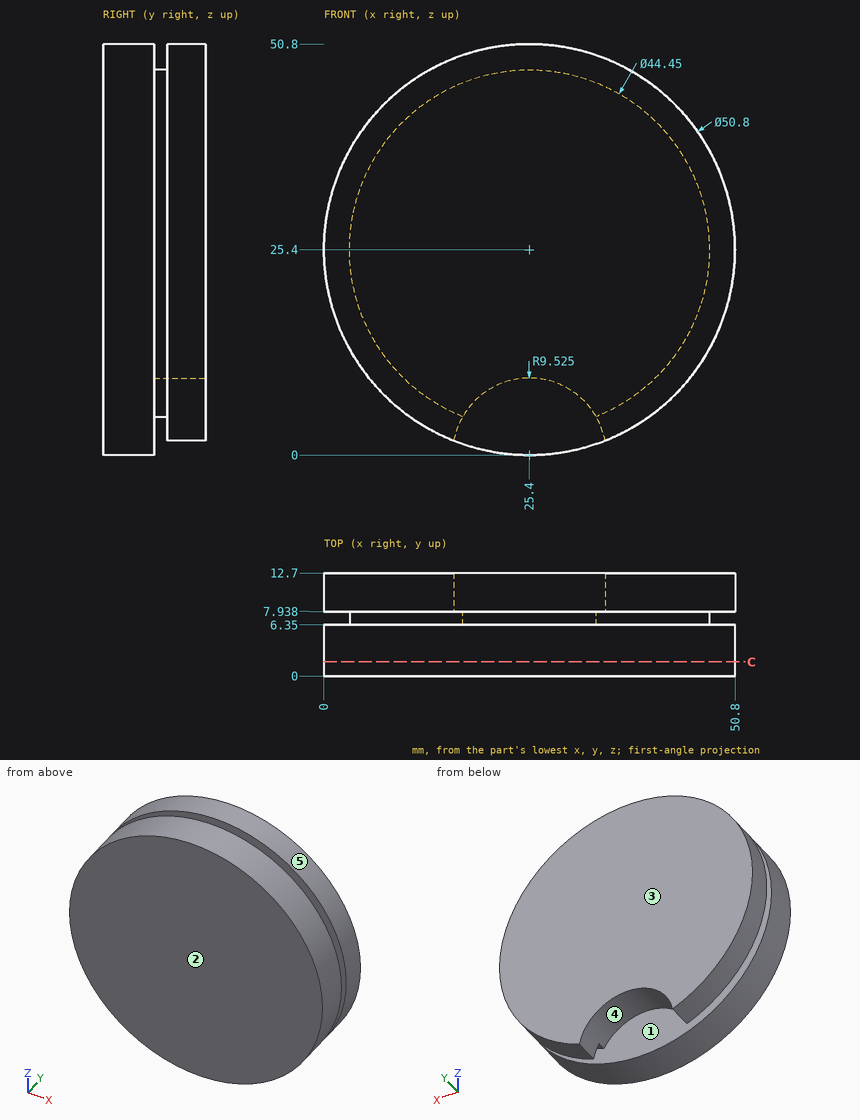
Geometry check sheet. Reference: drawing and pictorial views, mm from the part's lowest x, y, z. A direction names the side the tool comes from. Give positions to 0.01 mm unless a question says otherwise; leave off trailing zeros. Loops run counter-clockwise (first coordinate to the right, second up) from the corner with the lowest first, then second, coordinate; pieces in that order, holes last. Notation, with made-up numbers: M -26,40.25 L -9,40.25 A31 cw -9,68.25 Z; hole C 37,-25.75 d5. An arc over 180 degrees is marked long. One line per question, with ' | ' between items.
Item 1: Thickness scan on line 1 (Y direction, x = 19, z = 47); line 2 (Y direction, x = 22, z = 2); line 3 (Z direction, x = 44.5, y = 9.5) (1 decimal). Record the ranges inside material, lowest first. Write a range as [from, to].
Completed:
line 1: y = [0, 6.35], [7.94, 12.7] | line 2: y = [0, 6.35] | line 3: z = [8.7, 42.1]
Item 2: Draft check along X on the marked faces 3, 4 and 5. Enter one of: +X half, -X half, draft (parallel to the pull), parting line (faces both ways), or undercut.
Completed:
face 3: draft | face 4: undercut | face 5: parting line
Item 3: Tool access check on the marked faces 1 and 2. Record the directions out of +Z, -Z, +X, -X, +Y, -Y that give a thin tool (end or side, any length) a straight path to the whole face; none if there is none.
Completed:
face 1: none | face 2: +Z, -Z, +X, -X, -Y
Item 4: Depth check by flat-ended pin: P1, Ø1, axis at y = 4, z = 16.5, coming from the -X side; P2, Ø3, axis at y = 5.5, z = 20, coming from the +X side; P3, Ø3, axis at y = 3, z = 36, coming from the +X side (1 decimal). Enter the tip coordinate at first touch or a pass-through.
Completed:
P1: stops at x = 1.43 | P2: stops at x = 50.5 | P3: stops at x = 49.1
Item 5: Section check C-C, the plane y = 1.75. Record the cut outline in (x, z).
Completed:
outline: C 25.4,25.4 d50.8
